Check sheet for the modelled part. Datum: model origin and axes. Units: mm. A direction names the side the tool comes from. Round coordinates to 2 decimals unless told otherwise and drop trailing zeros. Write each loop counter-clockwise with the first axis right and the second up, starting at its lowest first coordinate (ties: lowest second). Pieces come first, ordered by that corner, then holes. Notation, with made-up numbers: (86.5, 23.5) -> (135.5, 23.5) arc R12 ccw to (135.5, 36.5) -> close; hole circle Ø3 at (67, 51). An arc over 180 degrees is marked (long way). Write item = value, one per line.
from build123d import *
from build123d.topology import SkipClean

# Parameters (mm, degrees)
SKETCH8_R               = 175
SKETCH8_R_2             = 125
BOSS_EXTRUDE7_DEPTH     = 50
SKETCH9_R               = 130
SKETCH9_R_2             = 125
CUT_EXTRUDE2_DEPTH      = 47.5
CUT_EXTRUDE3_DEPTH      = 267.926956301
CUT_EXTRUDE3_DEPTH_BACK = 267.926956301
SKETCH11_R              = 175
SKETCH11_R_2            = 125
BOSS_EXTRUDE8_DEPTH     = 2.5


with BuildPart() as part:
    # Sketch8 → Boss-Extrude7 (new, symmetric)
    with BuildSketch(Plane.YZ):
        with Locations(Location((0, 0, 0), (0, 0, 270))):
            Circle(SKETCH8_R)
        with Locations(Location((0, 0, 0), (0, 0, 270))):
            Circle(SKETCH8_R_2, mode=Mode.SUBTRACT)
    extrude(amount=BOSS_EXTRUDE7_DEPTH, both=True)

    # Sketch9 → Cut-Extrude2 (cut, symmetric)
    with BuildSketch(Plane.YZ):
        with Locations(Location((0, 0, 0), (0, 0, 270))):
            Circle(SKETCH9_R)
        with Locations(Location((0, 0, 0), (0, 0, 270))):
            Circle(SKETCH9_R_2, mode=Mode.SUBTRACT)
    extrude(amount=CUT_EXTRUDE2_DEPTH, both=True, mode=Mode.SUBTRACT)

    # Sketch10 → Cut-Extrude3 (cut, two sides: drawn at the far end of the back side and taken through both)
    with BuildSketch(Plane.YZ.offset(50).offset(-CUT_EXTRUDE3_DEPTH_BACK)):
        with BuildLine():
            Line((114.333214455, 71.783814835), (148.992574075, 91.794405442))
            ThreePointArc((148.992574075, 91.794405442), (87.5, 151.554445662), (5, 174.928556845))
            Line((5, 174.928556845), (5, 134.907375632))
            ThreePointArc((5, 134.907375632), (67.5, 116.913429511), (114.333214455, 71.783814835))
        make_face()
        with BuildLine():
            ThreePointArc((153.992574075, -83.134151404), (175, 0), (153.992574075, 83.134151404))
            Line((153.992574075, 83.134151404), (119.333214455, 63.123560797))
            ThreePointArc((119.333214455, 63.123560797), (135, 0), (119.333214455, -63.123560797))
            Line((119.333214455, -63.123560797), (153.992574075, -83.134151404))
        make_face()
        with BuildLine():
            ThreePointArc((-114.333214455, 71.783814835), (-67.5, 116.913429511), (-5, 134.907375632))
            Line((-5, 134.907375632), (-5, 174.928556845))
            ThreePointArc((-5, 174.928556845), (-87.5, 151.554445662), (-148.992574075, 91.794405442))
            Line((-148.992574075, 91.794405442), (-114.333214455, 71.783814835))
        make_face()
        with BuildLine():
            Line((148.992574075, -91.794405442), (114.333214455, -71.783814835))
            ThreePointArc((114.333214455, -71.783814835), (67.5, -116.913429511), (5, -134.907375632))
            Line((5, -134.907375632), (5, -174.928556845))
            ThreePointArc((5, -174.928556845), (87.5, -151.554445662), (148.992574075, -91.794405442))
        make_face()
        with BuildLine():
            ThreePointArc((-119.333214455, -63.123560797), (-135, 0), (-119.333214455, 63.123560797))
            Line((-119.333214455, 63.123560797), (-153.992574075, 83.134151404))
            ThreePointArc((-153.992574075, 83.134151404), (-175, 0), (-153.992574075, -83.134151404))
            Line((-153.992574075, -83.134151404), (-119.333214455, -63.123560797))
        make_face()
        with BuildLine():
            Line((-5, -174.928556845), (-5, -134.907375632))
            ThreePointArc((-5, -134.907375632), (-67.5, -116.913429511), (-114.333214455, -71.783814835))
            Line((-114.333214455, -71.783814835), (-148.992574075, -91.794405442))
            ThreePointArc((-148.992574075, -91.794405442), (-87.5, -151.554445662), (-5, -174.928556845))
        make_face()
    extrude(amount=CUT_EXTRUDE3_DEPTH + CUT_EXTRUDE3_DEPTH_BACK, mode=Mode.SUBTRACT)

    # Sketch11 → Boss-Extrude8 (add)
    with SkipClean():  # the faces are left unmerged after this step: merging them gives an invalid solid
        with BuildSketch(Plane.YZ.offset(50)):
            with Locations(Location((0, 0, 0), (0, 0, 88.362754922))):
                Circle(SKETCH11_R)
            with Locations(Location((0, 0, 0), (0, 0, 270))):
                Circle(SKETCH11_R_2, mode=Mode.SUBTRACT)
        boss_extrude8 = extrude(amount=-BOSS_EXTRUDE8_DEPTH)
    add(part.part.scale(1), mode=Mode.REPLACE)  # the faces are merged on a copy

    # Mirror3: Boss-Extrude8 across plane
    with SkipClean():  # the faces are left unmerged after this step: merging them gives an invalid solid
        add(boss_extrude8.mirror(Plane(origin=(0, 0, 0), x_dir=(0, 0, 1), z_dir=(1, 0, 0))))


solid = part.part
(1) Material ranges on L1, parallel to X at y = -138.5, z = 61; L2, parallel to Y at x = 14, z = 0; L3, parallel to Y at x = 18, z = 135, recorded low to high. Write a range as [from, to].
Worked answers:
L1 = [-50, -47.5], [47.5, 50]
L2 = [-135, -130], [130, 135]
L3 = [-5, 5]
(2) Sectioned sample at B-B on x = 40.5. Enter the section's corners in (y, z).
Worked answers:
outline = (-153.99, -83.13) arc R175 ccw to (-148.99, -91.79) -> (-114.33, -71.78) arc R135 ccw to (-5, -134.91) -> (-5, -174.93) arc R175 ccw to (5, -174.93) -> (5, -134.91) arc R135 ccw to (114.33, -71.78) -> (148.99, -91.79) arc R175 ccw to (153.99, -83.13) -> (119.33, -63.12) arc R135 ccw to (119.33, 63.12) -> (153.99, 83.13) arc R175 ccw to (148.99, 91.79) -> (114.33, 71.78) arc R135 ccw to (5, 134.91) -> (5, 174.93) arc R175 ccw to (-5, 174.93) -> (-5, 134.91) arc R135 ccw to (-114.33, 71.78) -> (-148.99, 91.79) arc R175 ccw to (-153.99, 83.13) -> (-119.33, 63.12) arc R135 ccw to (-119.33, -63.12) -> close; hole circle Ø260 at (0, 0)
(3) Sectioned sample at D-D on y = -65.5. Enter the section's corners in (x, z).
Worked answers:
outline = (-50, -162.28) -> (-47.5, -162.28) -> (-47.5, -118.05) -> (47.5, -118.05) -> (47.5, -162.28) -> (50, -162.28) -> (50, -106.46) -> (47.5, -106.46) -> (47.5, -112.29) -> (-47.5, -112.29) -> (-47.5, -106.46) -> (-50, -106.46) -> close; (-50, 106.46) -> (-47.5, 106.46) -> (-47.5, 112.29) -> (47.5, 112.29) -> (47.5, 106.46) -> (50, 106.46) -> (50, 162.28) -> (47.5, 162.28) -> (47.5, 118.05) -> (-47.5, 118.05) -> (-47.5, 162.28) -> (-50, 162.28) -> close
(4) Sectioned sample at A-A on y = 0. Enter the section's corners in (x, z), then the cut area to 3 significant figures.
Worked answers:
outline = (-50, -175) -> (50, -175) -> (50, -125) -> (47.5, -125) -> (47.5, -130) -> (-47.5, -130) -> (-47.5, -125) -> (-50, -125) -> close; (-50, 125) -> (-47.5, 125) -> (-47.5, 130) -> (47.5, 130) -> (47.5, 125) -> (50, 125) -> (50, 175) -> (-50, 175) -> close
area = 9,050 mm²
(5) Go/stop test with flat-tipped pins: P1, Ø20, axis at x = 10, z = 157, coming from the +Y side; P2, Ø1, axis at x = 14.5, y = 13.5, coming from the +Z side; P3, Ø2, axis at x = -6.5, y = -122, coming from the -Z side. Record where each tip stops, or that it passes through.
Worked answers:
P1 = 5
P2 = 134.37
P3 = -76.79
(6) Release check for a two-part mould opening along Z. For faces 6 (the flat face through (47.5, 152, -1)), 7 (the flat face through (-47.5, 107, 68)), 8 (the cylindrical face through (-0.665, -68.295, 116.451)), 9 (the flat face through (-1, 5, -155)) record: pulls with the +Z half, pulls with the -Z half, needs draft (parallel to the pull), parting line crosses it, or undercut.
Worked answers:
face_6 = undercut
face_7 = undercut
face_8 = pulls with the +Z half
face_9 = needs draft
(7) Access from +Z, -Z, +X, -X, +Y, -Y to the whole of each face (thin tool, end or side, straight path). Record for faces 1 (the flat face through (50, -120, -38)), 2 (the flat face through (-0.66, 131.91, -81.93)), 3 (the cylindrical face through (0.665, 39.048, -123.997)), 4 (the flat face through (-47.5, 152, -1)), 5 (the flat face through (-0.66, 131.42, 81.65)).
Worked answers:
face_1 = +Z, -Z, +X, +Y, -Y
face_2 = -Z
face_3 = none
face_4 = +Y
face_5 = +Z
(8) Sectioned sample at C-C on z = 18.5. Enter the section's corners in (x, y).
Worked answers:
outline = (-50, -174.02) -> (-47.5, -174.02) -> (-47.5, -133.73) -> (47.5, -133.73) -> (47.5, -174.02) -> (50, -174.02) -> (50, -123.62) -> (47.5, -123.62) -> (47.5, -128.68) -> (-47.5, -128.68) -> (-47.5, -123.62) -> (-50, -123.62) -> close; (-50, 123.62) -> (-47.5, 123.62) -> (-47.5, 128.68) -> (47.5, 128.68) -> (47.5, 123.62) -> (50, 123.62) -> (50, 174.02) -> (47.5, 174.02) -> (47.5, 133.73) -> (-47.5, 133.73) -> (-47.5, 174.02) -> (-50, 174.02) -> close
